Read the model definition and answer for the solid it produces. Units are mm, in the model's axes. A direction names the side the tool comes from. Coordinates: 2 decimals unless noted, no trailing zeros. Write each loop counter-clockwise with the first axis right and the second up, starting at its lowest first coordinate (ties: lowest second). Pieces come first, ordered by that corner, then holes.
(1) Section A-A on y = 0 is taken. Write down the section's boundary in (x, z), then the cut area to 3 significant figures.
(2) Which of the six approach directions +Z, -Z, +X, -X, +Y, -Y give full straight-line access (tool end or side, diameter ignored) to faces 4 (the cylindrical face through (-29.939, -7.615, 3.219)), 5 (the flat face through (-12.7, 0, 3))?
(3) Section C-C on z = 2.75 is taken. State how many separate pieces and enclosed holes the cut face has, then the cut area to 3 significant figures.
(4) Section D-D on y = 33 is taken. Write down the section's boundary in (x, z).
(5) Find the intervals of material crossed by probe 1 along Y at (x, z) = (0, 4) (1 decimal); probe 2 along Y at (x, z) = (13.16, 5.25) (3 decimals); probe 3 along X at (y, z) = (21, 4.25), in increasing order.
(6) Given pin 1 (2 mm diameter, centred on y = 31.5, z = 1, fed in from +X); pin 2 (0.9 mm diameter, centred on y = 28.5, z = 2.5, fed in from +X); pin 3 (3.5 mm diameter, centred on y = 28.5, z = 2.5, fed in from -X), each flat-ended and moving along its own axis, determine where each tip first touches the part or whether it passes through.
(7) Section B-B on x = 23.5 is taken. Write down the section's boundary in (y, z) (3 decimals).
(8) The mould has two halves that part along X. Classify faces 1 (the cylindrical face through (-24.36, 34.97, 3.13)), 2 (the flat face through (-25.4, 0, 3)), 3 (the cylindrical face through (29.84, -7.714, 3.219)): +X half, -X half, draft (parallel to the pull), parting line (faces both ways), or undercut.
from build123d import *

# Parameters (mm, degrees)
SKETCH1_W           = 63.5
SKETCH1_H           = 19.05
BOSS_EXTRUDE1_DEPTH = 6.35
SKETCH2_R           = 2.0955
SKETCH2_W           = 12.7
SKETCH2_H           = 6.35
CUT_EXTRUDE1_DEPTH  = 6.35
BOSS_EXTRUDE2_DEPTH = 6.35
SKETCH4_W           = 10
SKETCH4_H           = 3
CUT_EXTRUDE2_DEPTH  = 6.35
SKETCH5_R           = 8.336875
CUT_EXTRUDE3_DEPTH  = 6.35
SKETCH6_R           = 0.396875
CUT_EXTRUDE4_DEPTH  = 6.35
FILLET1_R           = 6.35


with BuildPart() as part:
    # Sketch1 → Boss-Extrude1 (new body)
    with BuildSketch(Plane.XY):
        Rectangle(SKETCH1_W, SKETCH1_H)
    extrude(amount=BOSS_EXTRUDE1_DEPTH)

    # Sketch2 → Cut-Extrude1 (cut)
    with BuildSketch(Plane.XY.offset(6.35)):
        Circle(SKETCH2_R)
        with Locations((-19.05, 0)):
            Rectangle(SKETCH2_W, SKETCH2_H)
        with Locations((19.05, 0)):
            Rectangle(SKETCH2_W, SKETCH2_H)
    extrude(amount=-CUT_EXTRUDE1_DEPTH, mode=Mode.SUBTRACT)

    # Sketch3 → Boss-Extrude2 (add)
    with BuildSketch(Plane.XY.offset(6.35)):
        Polygon((-31.75, 9.525), (-25.4, 36.375), (25.4, 36.375), (31.75, 9.525), align=None)
    extrude(amount=-BOSS_EXTRUDE2_DEPTH)

    # Sketch4 → Cut-Extrude2 (cut)
    with BuildSketch(Plane.XY.offset(6.35)):
        with BuildLine():
            Line((-3.25, 8.6375), (3.25, 8.6375))
            ThreePointArc((3.25, 8.6375), (6.0875, 11.475), (3.25, 14.3125))
            Line((3.25, 14.3125), (-3.25, 14.3125))
            ThreePointArc((-3.25, 14.3125), (-6.0875, 11.475), (-3.25, 8.6375))
        make_face()
        with Locations((0, 28.2025)):
            Rectangle(SKETCH4_W, SKETCH4_H)
    extrude(amount=-CUT_EXTRUDE2_DEPTH, mode=Mode.SUBTRACT)

    # Sketch5 → Cut-Extrude3 (cut)
    with BuildSketch(Plane.XY.offset(6.35)):
        with Locations((-12.34, 19.775)):
            Circle(SKETCH5_R)
        with Locations((13.16, 19.775)):
            Circle(SKETCH5_R)
    extrude(amount=-CUT_EXTRUDE3_DEPTH, mode=Mode.SUBTRACT)

    # Sketch6 → Cut-Extrude4 (cut)
    with BuildSketch(Plane(origin=(0, 0, 0), x_dir=(-1, 0, 0), z_dir=(0, 0, -1))):
        with Locations((20.45, 11.575)):
            Circle(SKETCH6_R)
        with Locations((-20.45, 27.975)):
            Circle(SKETCH6_R)
    extrude(amount=-CUT_EXTRUDE4_DEPTH, mode=Mode.SUBTRACT)

    # Fillet1
    fillet1_edges = [part.edges().sort_by_distance(p)[0] for p in [
        (-25.4, 36.375, 3.175),
        (25.4, 36.375, 3.175),
        (31.75, -9.525, 3.175),
        (-31.75, -9.525, 3.175),
        (-31.75, 9.525, 3.175),
        (31.75, 9.525, 3.175),
    ]]
    fillet(fillet1_edges, radius=FILLET1_R)


solid = part.part
Response:
1. outline: (-31.75, 0) - (-25.4, 0) - (-25.4, 6.35) - (-31.75, 6.35) - close; (-12.7, 0) - (-2.1, 0) - (-2.1, 6.35) - (-12.7, 6.35) - close; (2.1, 0) - (12.7, 0) - (12.7, 6.35) - (2.1, 6.35) - close; (25.4, 0) - (31.75, 0) - (31.75, 6.35) - (25.4, 6.35) - close
1. area: 215 mm2
2. face 4: +Z, -Z, -X, -Y
2. face 5: +Z, -Z
3. separate pieces: 1
3. enclosed holes: 9
3. area: 2,010 mm2
4. outline: (-25.99, 0) - (25.99, 0) - (25.99, 6.35) - (-25.99, 6.35) - close
5. probe 1: y = -9.5 to -2.1, 2.1 to 8.6, 14.3 to 26.7, 29.7 to 36.4
5. probe 2: y = -9.525 to -3.175, 3.175 to 11.438, 28.112 to 36.375
5. probe 3: x = -29.04 to -20.59, -4.09 to 4.91, 21.41 to 29.04
6. pin 1: stops at x = 26.79
6. pin 2: stops at x = 27.37
6. pin 3: stops at x = -27.68
7. outline: (-9.525, 0) - (-3.175, 0) - (-3.175, 6.35) - (-9.525, 6.35) - close; (3.175, 0) - (35.554, 0) - (35.554, 6.35) - (3.175, 6.35) - close
8. face 1: -X half
8. face 2: undercut
8. face 3: +X half
